Verification items for the finished model (mm, model axes). A direction names the side the tool comes from. Coordinates: 2 decimals unless noted, no trailing zeros. Order: outer loops, then holes, each group sorted by start corner. A loop starts at its lowest first (then second) coordinate and runs counter-clockwise, first axis right, second up.
Q1. Depth check by flat-ended pin: P1, Ø5.5, axis at x = -55.5, y = 4.5, coming from the +Z side; P2, Ø2, axis at x = -55, y = 5, coming from the -Z side. Enter the tip coordinate at first touch or a pass-through.
Q2. Set-up check for faces 1 (the cylindrical face through (54.241, 1.583, -0.986)), 2 (the cylindrical face through (0.38, 3.29, -3.01)): record each of +Z, -Z, +X, -X, +Y, -Y from which the full face is reachable in a straight line by a thin tool's end or side.
Q3. Draft check along Y on faces 3 (the flat face through (-1, 0, -2)), 4 (the cylindrical face through (-56.617, 4.33, -3.014)), 5 (the flat face through (75, 5, -2)). Enter one of: pulls with the +Y half, pulls with the -Y half, needs draft (parallel to the pull), parting line crosses it, or undercut.
Q4. Cross-section at A-A, the plane z = -3. Record the boundary of the cut face in (x, y).
Q5. Cross-section at B-B, the plane x = -55. Record the boundary of the cut face in (y, z), and give its area (3 significant figures).
Q6. Thickness scan on line 1 (X direction, y = 4.75, z = -1.3); line 2 (X direction, y = 3.75, z = -1.4); line 3 (Y direction, x = 0, z = -3.2). Record the ranges inside material, lowest first.
Q7. Cross-section at C-C, the plane x = 33.5. Record the boundary of the cut face in (y, z).
from build123d import *

# Parameters (mm, degrees)
F0_W           = 150
F0_H           = 10
F1_DEPTH       = 4
F2_D           = 3.5
F2_CBORE_D     = 7
F2_CBORE_DEPTH = 2
F3_T1_DEPTH    = 160.2867319519


# Not quite as in the source:
# - a fillet or chamfer that OpenCascade refuses, or shapes differently, is made with other operations: its cross-section is extruded or revolved along the edge and cut away or added


with BuildPart() as f1:
    # F0 (on Top) → F1 (new body)
    with BuildSketch(Plane.XY):
        with Locations((0, 5)):
            Rectangle(F0_W, F0_H)
    extrude(amount=-F1_DEPTH)

    # F2 (through all)
    with Locations(Plane.XY):
        with Locations((-55, 5), (0, 5), (55, 5)):
            CounterBoreHole(F2_D / 2, F2_CBORE_D / 2, F2_CBORE_DEPTH)

    # F3: chamfer of 2 on 1 edges, made by hand

    # F3_s2 → F3_t1 (cut)
    with BuildSketch(Plane.YZ.offset(-80.1433659759)):
        Polygon((10, -2), (8, 0), (10, 0), align=None)
    extrude(amount=F3_T1_DEPTH, mode=Mode.SUBTRACT)


solid = f1.part
Check values:
1. P1: stops at z = -2
1. P2: passes through
2. face 1: +Z
2. face 2: +Z, -Z
3. face 3: pulls with the -Y half
3. face 4: undercut
3. face 5: needs draft
4. outline: (-75, 0) - (75, 0) - (75, 10) - (-75, 10) - close; hole circle Ø3.5 at (-55, 5); hole circle Ø3.5 at (0, 5); hole circle Ø3.5 at (55, 5)
5. outline: (0, -4) - (3.25, -4) - (3.25, -2) - (1.5, -2) - (1.5, 0) - (0, 0) - close; (6.75, -4) - (10, -4) - (10, -2) - (8.5, -0.5) - (8.5, -2) - (6.75, -2) - close
5. area: 17.1 mm2
6. line 1: x = -75 to -58.49, -51.51 to -3.49, 3.49 to 51.51, 58.49 to 75
6. line 2: x = -75 to -58.27, -51.73 to -3.27, 3.27 to 51.73, 58.27 to 75
6. line 3: y = 0 to 3.25, 6.75 to 10
7. outline: (0, -4) - (10, -4) - (10, -2) - (8, 0) - (0, 0) - close
